The model under review builds one solid part; all positions refer to its coordinate system, in mm. Face numbers are marked on the shaded views. Coordinates: 2 decimals unless noted, no trailing zeros. Write each loop counter-clockwise with the first axis right and the second up, starting at its lowest first coordinate (ties: lowest second). Pieces come first, ordered by that corner, then holes. Notation, with made-up numbers: (42.25, -22.5) - (66.25, -22.5) arc R15 cw to (66.25, -9.5) - close; hole circle Ø11 at (-31.75, 82.5). An arc over 180 degrees is marked (long way). Put each result on its own line as item: value. Start each with the question number.
Item 1: Mouldability with a two-part tool opening along Z and no side actions: class the marked faces 1 and 2 as pulls with the +Z half, pulls with the -Z half, needs draft (parallel to the pull), parting line crosses it, or undercut.
Item 2: To check wall thickness, follow L1, parallel to Y at x = 3, z = 1.5; L2, parallel to X at y = -5.25, z = 0.5; L3, parallel to Y at x = 17.5, z = 0.95. State the ranges of each line that lie inside material, in increasing order. Write a range as [from, to].
Item 3: Consider section C-C on z = 1.3. State how many separate pieces and enclosed holes the cut face has, then the cut area to 3 significant figures.
Item 4: For pin 1 (1.6 mm diameter, centred on x = 2.99, y = -9, fed in from -Z); pin 2 (0.6 mm diameter, centred on x = 48.5, z = 1, fed in from -Y); pin 3 (0.6 mm diameter, centred on x = 47.5, z = 1, fed in from +Y); pin 4 (1 mm diameter, centred on y = 9.5, z = 0.5, fed in from +X), all flat-tipped, find the tip position at first contact; note any pin that passes through.
Item 5: Consider section A-A on y = -2.25. Give the boundary of the cut face in (x, z), then the cut area to 3 significant figures.
Item 6: Consider section B-B on x = 44. Give the boundary of the cut face in (y, z), then the cut area to 3 significant figures.
```python
from build123d import *

# Parameters (mm, degrees)
BOSS_EXTRU_1_OUTLINE_W   = 2
BOSS_EXTRU_1_OUTLINE_H   = 5
BOSS_EXTRU_1_OUTLINE_R   = 1
BOSS_EXTRU_1_OUTLINE_R_2 = 1.5
BOSS_EXTRU_1_DEPTH       = 2
FILLET1_R                = 4


# Read off the part's stored shape, not the designer's step: Boss.-Extru.1
with BuildPart() as part:
    # Boss.-Extru.1 outline → Boss.-Extru.1 (new body)
    with BuildSketch(Plane.XY):
        Polygon((-7, -14.16114291), (31, -14.16114291), (51, -12.5), (51, 12.5), (31, 14.16114291), (-7, 14.16114291), align=None)
        with Locations((-3.924802108, -7.5)):
            Rectangle(BOSS_EXTRU_1_OUTLINE_W, BOSS_EXTRU_1_OUTLINE_H, mode=Mode.SUBTRACT)
        with Locations((2.98759897, -9.000034515)):
            Circle(BOSS_EXTRU_1_OUTLINE_R, mode=Mode.SUBTRACT)
        with Locations((31.315776387, -9.000034515)):
            Circle(BOSS_EXTRU_1_OUTLINE_R, mode=Mode.SUBTRACT)
        with Locations((41.98759897, -9.000034515)):
            Circle(BOSS_EXTRU_1_OUTLINE_R, mode=Mode.SUBTRACT)
        with Locations((47.975197892, -7.5)):
            Rectangle(BOSS_EXTRU_1_OUTLINE_W, BOSS_EXTRU_1_OUTLINE_H, mode=Mode.SUBTRACT)
        with BuildLine():
            ThreePointArc((33.615776345, -8.000034132), (33.23501504, -7.080795537), (32.315776344, -6.700034473))
            Line((32.315776344, -6.700034473), (30.315776345, -6.700034473))
            ThreePointArc((30.315776345, -6.700034473), (29.396536008, -7.080797161), (29.015776303, -8.000038733))
            Line((29.015776303, -8.000038733), (29.015776303, -12.100034515))
            Line((29.015776303, -12.100034515), (5.28759897, -12.100034515))
            Line((5.28759897, -12.100034515), (5.28759897, -7.950034515))
            ThreePointArc((5.28759897, -7.950034515), (4.921479782, -7.066148374), (4.037591434, -6.700034515))
            Line((4.037591434, -6.700034515), (0, -6.699965485))
            Line((0, -6.699965485), (0, 6.699965485))
            Line((0, 6.699965485), (4.03758425, 6.699965485))
            ThreePointArc((4.03758425, 6.699965485), (4.921477242, 7.066076805), (5.28759897, 7.949965485))
            Line((5.28759897, 7.949965485), (5.28759897, 11.987564455))
            Line((5.28759897, 11.987564455), (29.015776399, 11.987564455))
            Line((29.015776399, 11.987564455), (29.015776399, 7.999965373))
            ThreePointArc((29.015776399, 7.999965373), (29.396537621, 7.080726637), (30.31577639, 6.699965495))
            Line((30.31577639, 6.699965495), (32.315776389, 6.699965495))
            ThreePointArc((32.315776389, 6.699965495), (33.235016597, 7.080728053), (33.615776432, 7.999969389))
            Line((33.615776432, 7.999969389), (33.615776432, 11.987564455))
            Line((33.615776432, 11.987564455), (39.68759897, 11.987564455))
            Line((39.68759897, 11.987564455), (39.68759897, 7.949965701))
            ThreePointArc((39.68759897, 7.949965701), (40.053716981, 7.066080502), (40.9376034, 6.699965437))
            Line((40.9376034, 6.699965437), (44.975197892, 6.699965437))
            Line((44.975197892, 6.699965437), (44.975197892, -6.70003437))
            Line((44.975197892, -6.70003437), (40.937599481, -6.70003437))
            ThreePointArc((40.937599481, -6.70003437), (40.053713738, -7.066152541), (39.687598777, -7.950039613))
            Line((39.687598777, -7.950039613), (39.687598777, -12.100034515))
            Line((39.687598777, -12.100034515), (33.615776345, -12.100034515))
            Line((33.615776345, -12.100034515), (33.615776345, -8.000034132))
        make_face(mode=Mode.SUBTRACT)
        with Locations((-3.924802108, 0)):
            Circle(BOSS_EXTRU_1_OUTLINE_R_2, mode=Mode.SUBTRACT)
        with Locations((-3.924802108, 7.5)):
            Rectangle(BOSS_EXTRU_1_OUTLINE_W, BOSS_EXTRU_1_OUTLINE_H, mode=Mode.SUBTRACT)
        with Locations((2.98759897, 8.999965485)):
            Circle(BOSS_EXTRU_1_OUTLINE_R, mode=Mode.SUBTRACT)
        with Locations((47.975197892, 0)):
            Circle(BOSS_EXTRU_1_OUTLINE_R_2, mode=Mode.SUBTRACT)
        with Locations((31.315776387, 8.999965485)):
            Circle(BOSS_EXTRU_1_OUTLINE_R, mode=Mode.SUBTRACT)
        with Locations((41.98759897, 8.999965485)):
            Circle(BOSS_EXTRU_1_OUTLINE_R, mode=Mode.SUBTRACT)
        with Locations((47.975197892, 7.5)):
            Rectangle(BOSS_EXTRU_1_OUTLINE_W, BOSS_EXTRU_1_OUTLINE_H, mode=Mode.SUBTRACT)
    extrude(amount=BOSS_EXTRU_1_DEPTH)

    # Fillet1
    # the kernel refuses this fillet: 4 mm, written as the material it takes off along each edge
    with BuildSketch(Plane(origin=(31, -14.16114291, -0.414571976), x_dir=(-1, 0, 0), z_dir=(0, 0, 1)), Plane(origin=(31, 14.16114291, -0.414571976), x_dir=(0.9965684992480803, -0.0827721348427634, 0), z_dir=(0, 0, 1))) as fillet1_piece_1:
        with BuildLine():
            CenterArc((FILLET1_R * 0.0414571976238, -FILLET1_R), FILLET1_R, 90, 4.747926068)
            Line((-FILLET1_R * 0.041314937219, -FILLET1_R * 0.00343150075192), (0, 0))
            Line((0, 0), (FILLET1_R * 0.0414571976238, 0))
        make_face()
    extrude(amount=2.829143952, mode=Mode.SUBTRACT)
    with BuildSketch(Plane(origin=(-7, -14.16114291, -10), x_dir=(1, 0, 0), z_dir=(0, 0, 1))) as fillet1_piece_2:
        with BuildLine():
            CenterArc((FILLET1_R, FILLET1_R), FILLET1_R, 180, 90)
            Line((0, FILLET1_R), (0, 0))
            Line((0, 0), (FILLET1_R, 0))
        make_face()
    extrude(amount=22, mode=Mode.SUBTRACT)
    with BuildSketch(Plane(origin=(-7, 14.16114291, -10), x_dir=(1, 0, 0), z_dir=(0, 0, 1))) as fillet1_piece_3:
        with BuildLine():
            CenterArc((FILLET1_R, -FILLET1_R), FILLET1_R, 90, 90)
            Line((0, -FILLET1_R), (0, 0))
            Line((0, 0), (FILLET1_R, 0))
        make_face()
    extrude(amount=22, mode=Mode.SUBTRACT)
    with BuildSketch(Plane(origin=(51, 12.5, -9.20386171), x_dir=(0, -1, 0), z_dir=(0, 0, 1)), Plane(origin=(51, -12.5, -9.20386171), x_dir=(-0.9965684992480804, -0.08277213484276448, 0), z_dir=(0, 0, 1))) as fillet1_piece_4:
        with BuildLine():
            CenterArc((FILLET1_R * 0.920386170995, -FILLET1_R), FILLET1_R, 90, 85.252073932)
            Line((-FILLET1_R * 0.076182328253, -FILLET1_R * 0.917227865157), (0, 0))
            Line((0, 0), (FILLET1_R * 0.920386170995, 0))
        make_face()
    extrude(amount=20.40772342, mode=Mode.SUBTRACT)


solid = part.part
```
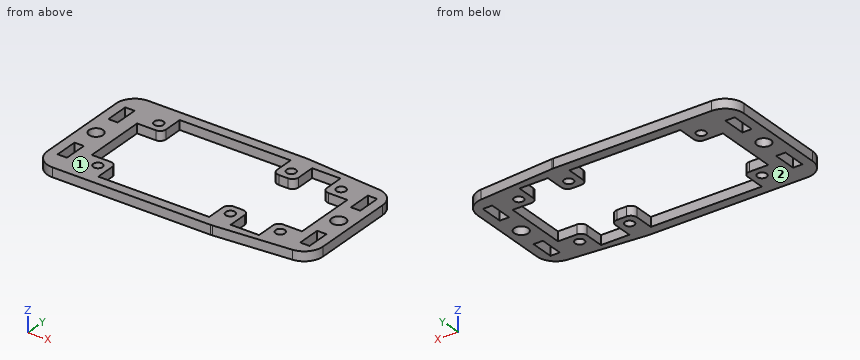
Report:
1. face 1: pulls with the +Z half
1. face 2: pulls with the -Z half
2. L1: [-14.16, -10], [-8, -6.7], [6.7, 8], [10, 14.16]
2. L2: [-7, -4.92], [-2.92, 0], [44.98, 46.98], [48.98, 51]
2. L3: [-14.16, -12.1], [11.99, 14.16]
3. separate pieces: 1
3. enclosed holes: 13
3. area: 600 mm²
4. pin 1: through
4. pin 2: y = -12.63
4. pin 3: y = 12.82
4. pin 4: x = 51
5. outline: (-7, 0) - (0, 0) - (0, 2) - (-7, 2) - close; (44.98, 0) - (51, 0) - (51, 2) - (44.98, 2) - close
5. area: 26.0 mm²
6. outline: (-13.08, 0) - (-6.7, 0) - (-6.7, 2) - (-13.08, 2) - close; (6.7, 0) - (13.08, 0) - (13.08, 2) - (6.7, 2) - close
6. area: 25.5 mm²
